Print and shaded views of the part. All mm, measured from the part's lowest x, y and z. A direction names the side the tool comes from. Round coordinates to 2 decimals unless told otherwise and drop trailing zeros. Loops run counter-clockwise (first coordinate to the right, second up) from the corner with the lowest first, then second, coordinate; pieces in that order, holes last. Notation, with made-up numbers: (25, 27.5) - (41, 27.5) arc R12 cw to (41, 46.5) - close; hole circle Ø1 at (41, -37.5). An arc over 180 degrees is marked (long way). Answer as a JSON object with one key per item and string values.
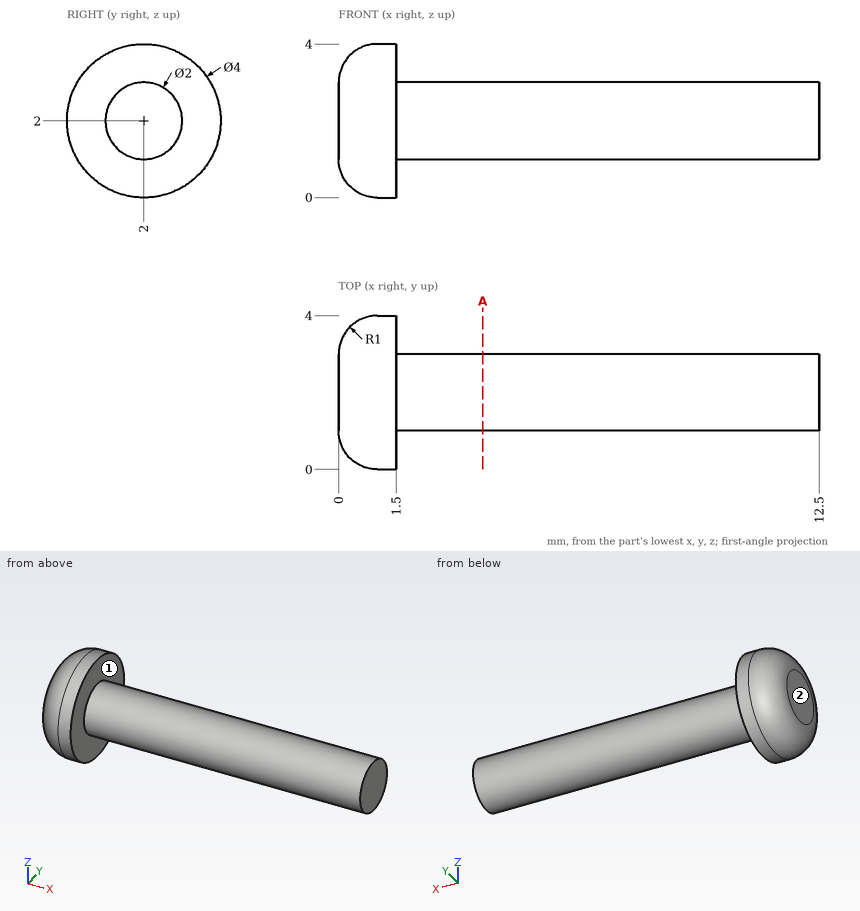
1) Slice it at A-A on x = 3.75. List the corners of the cut face in (y, z).
Values follow:
{"outline": "circle Ø2 at (2, 2)"}
2) Probe probe 1 along Y at (x, z) = (8.25, 2.4); probe 2 along Y at (x, z) = (9.25, 2.15); probe 3 along X at (y, z) = (0.5, 1.85). List the from-to ranges inside material, lowest first.
Values follow:
{"probe 1": "1.08 to 2.92", "probe 2": "1.01 to 2.99", "probe 3": "0.14 to 1.5"}
3) Tool access for the marked faces 1 and 2: list every direction of +Z, -Z, +X, -X, +Y, -Y with a clear straight run to the whole face (end or side of a thin tool).
Values follow:
{"face 1": "+X", "face 2": "+Z, -Z, -X, +Y, -Y"}
